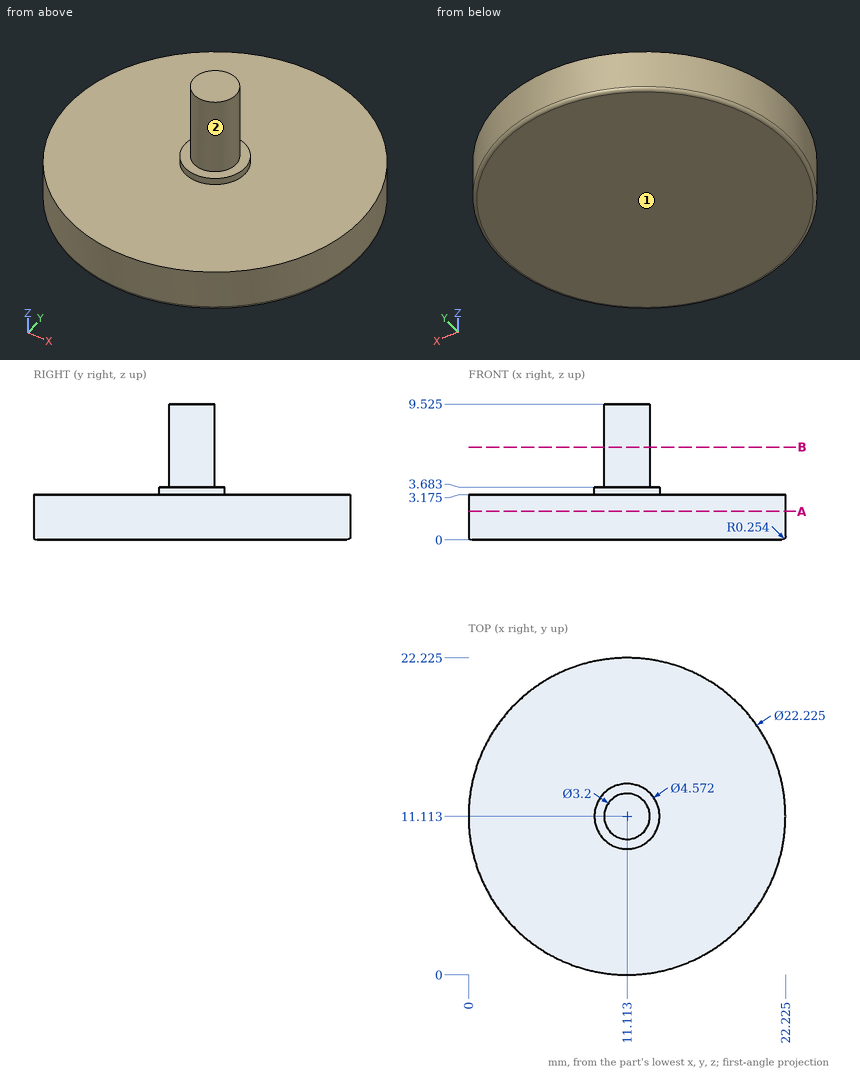
Geometry: see drawing. Coordinates: mm, zero at the bounding-box minimum. A direction names the side the tool comes from. Give positions to 0.01 mm unless a question says otherwise; leave off trailing zeros. Write each loop counter-clockwise with the first axis right and the second up, starting at its lowest first coordinate (ties: lowest second). Pieces come first, ordered by that corner, then holes. Notation, with made-up numbers: (62.25, -40) - (103.25, -40) arc R19 cw to (103.25, -16) - close; hole circle Ø1 at (66.25, 78). An arc over 180 degrees is marked (long way). Return JSON: item names as keys, results as strings. Group by question number.
1) Set-up query: the marked faces 1 and 2. Return all of +Z, -Z, +X, -X, +Y, -Y with unobstructed straight access to the full face (end or side cutting, diameter ignored); none if empty.
2) First-contact query: P1, Ø4, axis at y = 18, z = 6, coming from the +X side; P2, Ø1.5, axis at x = 6, z = 3, coming from the +Y side; P3, Ø6.5, axis at x = 13.5, y = 16.5, coming from the +Z side (1 decimal); P4, Ø3, axis at x = 9, z = 6.5, coming from the -Y side (1 decimal). Flat tips, straight axial feed; report the tip coordinate or a pass-through.
3) Section B-B on z = 6.5. Return the cut outline in (x, y).
4) Section A-A on z = 2. Return the cut outline in (x, y) (1 decimal).
5) Line query: line 1 (Z direction, x = 8.75, y = 16) (1 decimal); line 2 (Y direction, x = 11.75, z = 1); line 3 (X direction, y = 10.25, z = 3). Output: solid intervals per line, ascending.
Filled in:
{
 "1": {"face 1": "-Z, +X, -X, +Y, -Y", "face 2": "+Z"},
 "2": {"P1": "passes through", "P2": "stops at y = 21.33", "P3": "stops at z = 3.2", "P4": "stops at y = 9.6"},
 "3": {"outline": "circle Ø3.2 at (11.11, 11.11)"},
 "4": {"outline": "circle Ø22.2 at (11.1, 11.1)"},
 "5": {"line 1": "z = 0 to 3.2", "line 2": "y = 0.02 to 22.21", "line 3": "x = 0.03 to 22.19"}
}
